Here's how the part is built. I have some questions about the finished solid (model axes, mm). Coordinates: 2 decimals unless noted, no trailing zeros. Write each loop counter-clockwise with the first axis right and the second up, starting at its lowest first coordinate (ties: lowest second). Pieces come first, ordered by that corner, then holes.
(1) Imagine slicing it at C-C, the plane z = -200. List the corners of the cut face in (x, y) for me, plus the area to 3 significant figures.
(2) Imagine slicing it at B-B, the plane x = 332. List the corners of the cut face in (y, z) for me, plus the area to 3 significant figures.
(3) Please list where these lines run through material, in increasing order: probe 1 along X at (y, z) = (2.3, -580); probe 2 along Z at (x, y) = (580, 1.25); probe 3 along X at (y, z) = (1.65, -544).
(4) For pin 1 Ø3 at (y, z) = (20.5, -76.5) entering from +X; pin 2 Ø12 at (y, z) = (15, -431.5) entering from -X; pin 3 Ø1 at (x, z) = (82.5, -248.5) entering from +Y, each with a flat end and sliding along its axis, tell me the tip position at first contact or that it passes through.
(5) Imagine slicing it at A-A, the plane y = 22.5. State how many separate pieces and enclosed holes the cut face has, plus the area to 3 significant figures.
```python
from build123d import *

# Parameters (mm, degrees)
SKETCH1_W           = 600
SKETCH1_H           = 600
BOSS_EXTRUDE1_DEPTH = 4
CUT_EXTRUDE1_REACH  = 850.538
SKETCH2_R           = 4.5
CUT_EXTRUDE2_REACH  = 850.538
SKETCH4_R           = 3.25
SKETCH4_3_W         = 50
SKETCH4_3_H         = 6
SKETCH4_3_W_2       = 6
SKETCH4_3_H_2       = 40
BOSS_EXTRUDE2_DEPTH = 35
SKETCH5_W           = 6
SKETCH5_H           = 26.8
SKETCH5_W_2         = 26.8
SKETCH5_H_2         = 6
BOSS_EXTRUDE3_DEPTH = 35


with BuildPart() as part:
    # Sketch1 → Boss-Extrude1 (new body)
    with BuildSketch(Plane(origin=(0, 0, 0), x_dir=(1, 0, 0), z_dir=(0, 1, 0))):
        with Locations((300, 300)):
            Rectangle(SKETCH1_W, SKETCH1_H)
    extrude(amount=BOSS_EXTRUDE1_DEPTH)

    # Sketch2 → Cut-Extrude1 (cut, up to next)
    with BuildSketch(Plane(origin=(0, 4, 0), x_dir=(1, 0, 0), z_dir=(0, 1, 0)), mode=Mode.PRIVATE) as cut_extrude1_sk1:
        with Locations(Location((20, 580, 0), (0, 0, 270))):
            Circle(SKETCH2_R)
    cut_extrude1_tool1 = extrude(cut_extrude1_sk1.sketch, amount=-CUT_EXTRUDE1_REACH, mode=Mode.PRIVATE) & part.part
    # Sketch2 → Cut-Extrude1 (cut, up to next)
    with BuildSketch(Plane(origin=(0, 4, 0), x_dir=(1, 0, 0), z_dir=(0, 1, 0)), mode=Mode.PRIVATE) as cut_extrude1_sk2:
        with Locations(Location((580, 580, 0), (0, 0, 270))):
            Circle(SKETCH2_R)
    cut_extrude1_tool2 = extrude(cut_extrude1_sk2.sketch, amount=-CUT_EXTRUDE1_REACH, mode=Mode.PRIVATE) & part.part
    # Sketch2 → Cut-Extrude1 (cut, up to next)
    with BuildSketch(Plane(origin=(0, 4, 0), x_dir=(1, 0, 0), z_dir=(0, 1, 0)), mode=Mode.PRIVATE) as cut_extrude1_sk3:
        with Locations(Location((580, 20, 0), (0, 0, 270))):
            Circle(SKETCH2_R)
    cut_extrude1_tool3 = extrude(cut_extrude1_sk3.sketch, amount=-CUT_EXTRUDE1_REACH, mode=Mode.PRIVATE) & part.part
    # Sketch2 → Cut-Extrude1 (cut, up to next)
    with BuildSketch(Plane(origin=(0, 4, 0), x_dir=(1, 0, 0), z_dir=(0, 1, 0)), mode=Mode.PRIVATE) as cut_extrude1_sk4:
        with Locations(Location((20, 20, 0), (0, 0, 270))):
            Circle(SKETCH2_R)
    cut_extrude1_tool4 = extrude(cut_extrude1_sk4.sketch, amount=-CUT_EXTRUDE1_REACH, mode=Mode.PRIVATE) & part.part
    add(cut_extrude1_tool1.solids().sort_by_distance((20, 4, -580))[0], mode=Mode.SUBTRACT)
    add(cut_extrude1_tool2.solids().sort_by_distance((580, 4, -580))[0], mode=Mode.SUBTRACT)
    add(cut_extrude1_tool3.solids().sort_by_distance((580, 4, -20))[0], mode=Mode.SUBTRACT)
    add(cut_extrude1_tool4.solids().sort_by_distance((20, 4, -20))[0], mode=Mode.SUBTRACT)

    # Sketch4 → Cut-Extrude2 (cut, up to next)
    with BuildSketch(Plane(origin=(0, 4, 0), x_dir=(1, 0, 0), z_dir=(0, 1, 0)), mode=Mode.PRIVATE) as cut_extrude2_sk1:
        with Locations(Location((45.75, 544, 0), (0, 0, 270))):
            Circle(SKETCH4_R)
    cut_extrude2_tool1 = extrude(cut_extrude2_sk1.sketch, amount=-CUT_EXTRUDE2_REACH, mode=Mode.PRIVATE) & part.part
    # Sketch4 → Cut-Extrude2 (cut, up to next)
    with BuildSketch(Plane(origin=(0, 4, 0), x_dir=(1, 0, 0), z_dir=(0, 1, 0)), mode=Mode.PRIVATE) as cut_extrude2_sk2:
        with Locations(Location((45.75, 436, 0), (0, 0, 270))):
            Circle(SKETCH4_R)
    cut_extrude2_tool2 = extrude(cut_extrude2_sk2.sketch, amount=-CUT_EXTRUDE2_REACH, mode=Mode.PRIVATE) & part.part
    # Sketch4 → Cut-Extrude2 (cut, up to next)
    with BuildSketch(Plane(origin=(0, 4, 0), x_dir=(1, 0, 0), z_dir=(0, 1, 0)), mode=Mode.PRIVATE) as cut_extrude2_sk3:
        with Locations(Location((203.75, 436, 0), (0, 0, 270))):
            Circle(SKETCH4_R)
    cut_extrude2_tool3 = extrude(cut_extrude2_sk3.sketch, amount=-CUT_EXTRUDE2_REACH, mode=Mode.PRIVATE) & part.part
    # Sketch4 → Cut-Extrude2 (cut, up to next)
    with BuildSketch(Plane(origin=(0, 4, 0), x_dir=(1, 0, 0), z_dir=(0, 1, 0)), mode=Mode.PRIVATE) as cut_extrude2_sk4:
        with Locations(Location((203.75, 544, 0), (0, 0, 270))):
            Circle(SKETCH4_R)
    cut_extrude2_tool4 = extrude(cut_extrude2_sk4.sketch, amount=-CUT_EXTRUDE2_REACH, mode=Mode.PRIVATE) & part.part
    add(cut_extrude2_tool1.solids().sort_by_distance((45.75, 4, -544))[0], mode=Mode.SUBTRACT)
    add(cut_extrude2_tool2.solids().sort_by_distance((45.75, 4, -436))[0], mode=Mode.SUBTRACT)
    add(cut_extrude2_tool3.solids().sort_by_distance((203.75, 4, -436))[0], mode=Mode.SUBTRACT)
    add(cut_extrude2_tool4.solids().sort_by_distance((203.75, 4, -544))[0], mode=Mode.SUBTRACT)

    # Sketch4_3 → Boss-Extrude2 (add)
    with BuildSketch(Plane(origin=(0, 4, 0), x_dir=(1, 0, 0), z_dir=(0, 1, 0))):
        with Locations((124.75, 553)):
            Rectangle(SKETCH4_3_W, SKETCH4_3_H)
        with Locations((37, 490)):
            Rectangle(SKETCH4_3_W_2, SKETCH4_3_H_2)
        with Locations((212.5, 490)):
            Rectangle(SKETCH4_3_W_2, SKETCH4_3_H_2)
        with Locations((124.75, 427)):
            Rectangle(SKETCH4_3_W, SKETCH4_3_H)
    extrude(amount=BOSS_EXTRUDE2_DEPTH)

    # Sketch5 → Boss-Extrude3 (add)
    with BuildSketch(Plane(origin=(0, 4, 0), x_dir=(1, 0, 0), z_dir=(0, 1, 0))):
        with Locations((71, 250.6)):
            Rectangle(SKETCH5_W, SKETCH5_H)
        with Locations((468.6, 277)):
            Rectangle(SKETCH5_W_2, SKETCH5_H_2)
        with Locations((495, 250.6)):
            Rectangle(SKETCH5_W, SKETCH5_H)
        with Locations((495, 103.4)):
            Rectangle(SKETCH5_W, SKETCH5_H)
        with Locations((468.6, 77)):
            Rectangle(SKETCH5_W_2, SKETCH5_H_2)
        with Locations((97.4, 277)):
            Rectangle(SKETCH5_W_2, SKETCH5_H_2)
        with Locations((71, 103.4)):
            Rectangle(SKETCH5_W, SKETCH5_H)
        with Locations((97.4, 77)):
            Rectangle(SKETCH5_W_2, SKETCH5_H_2)
    extrude(amount=BOSS_EXTRUDE3_DEPTH)


solid = part.part
```
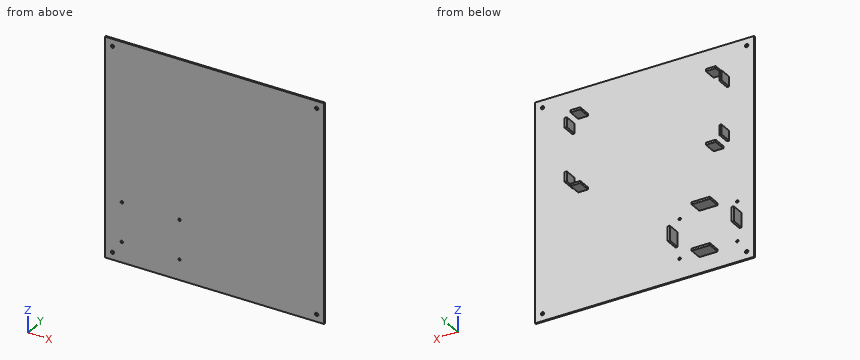
Recorded:
1. outline: (0, 0) - (600, 0) - (600, 4) - (0, 4) - close
1. area: 2,400 mm2
2. outline: (0, -600) - (4, -600) - (4, 0) - (0, 0) - close
2. area: 2,400 mm2
3. probe 1: x = 0 to 15.5, 24.5 to 575.5, 584.5 to 600
3. probe 2: z = -600 to -584.5, -575.5 to -24.5, -15.5 to 0
3. probe 3: x = 0 to 42.5, 49 to 200.5, 207 to 600
4. pin 1: stops at x = 482
4. pin 2: stops at x = 99.75
4. pin 3: stops at y = 4
5. separate pieces: 12
5. enclosed holes: 0
5. area: 2,370 mm2
